Input: part model. Units: mm. Frame: model coordinates. A direction names the side the tool comes from. Coordinates: 2 decimals unless noted, no trailing zeros. Order: outer loops, then holes, each group sorted by start corner. A loop starts at its lowest first (then second) coordinate and runs counter-clockwise, first axis right, second up. Notation, with made-up numbers: M 15,52.25 L 61,52.25 A32 cw 61,81.25 Z; hole C -3.5,69.5 d4. An arc over 180 degrees is marked long. One line per item, written item: value.
Autodesk Inventor part; units mm, degrees
ref_plane "YZ Plane" through (0, 0, 0) normal (1, 0, 0) x (0, 1, 0)
ref_plane "XZ Plane" through (0, 0, 0) normal (0, 1, 0) x (-1, 0, 0)
ref_plane "XY Plane" through (0, 0, 0) normal (0, 0, 1) x (1, 0, 0)
sketch "Skizze1" plane through (0, 0, 0) normal (0, 0, 1) x (1, 0, 0)
  circle A0 centre (0, 0) radius 11.1 construction
  circle A1 centre (0, 0) radius 25
  circle A2 centre (0, 0) radius 15
  circle A3 centre (-15, -15) radius 1.25
  circle A4 centre (15, 15) radius 1.25
  circle A5 centre (15, -15) radius 1.25
  circle A6 centre (-15, 15) radius 1.25
  point P0 (0, 0)
  dimension "d0" = 30
extrude "Extrusion1" add sketch "Skizze1" along normal blind 9 contours A1 | A3 | A4 | A5 | A6
sketch "Skizze2" plane through (0, 0, 9) normal (0, 0, 1) x (1, 0, 0)
  circle A0 centre (0, 0) radius 15
  circle A1 centre (0, 0) radius 25
  point P0 (0, 0)
extrude "Extrusion2" add sketch "Skizze2" against normal blind 2 contours A0
fillet "Rundung1" radius 5 1 edges at (-25, 0, 9)
sketch "Skizze3" plane through (0, 0, 9) normal (0, 0, 1) x (1, 0, 0)
  line L0 (-15, -15) -> (15, -15)
  line L1 (15, -15) -> (15, 15)
  line L2 (15, 15) -> (-15, 15)
  line L3 (-15, 15) -> (-15, -15)
  line L4 (-15, -15) -> (15, 15) construction
  line L5 (15, -15) -> (-15, 15) construction
  point P0 (0, 0)
  dimension "d6" = 30
hole "Bohrung1" at (-15, 15, 9) at (15, 15, 9) at (15, -15, 9) at (-15, -15, 9) direction (0, 0, -1) diameter 3 depth 8 tip angle 118 counterbore diameter 6 counterbore depth 4
properties part number "Cover_G2" material "ABS-Kunststoff"
(1) Cut plane A-A on x = 0. Output: boundary loops of the cut face in (y, z).
Data:
outline: M -25,0 L -15,0 L -15,7 L 15,7 L 15,0 L 25,0 L 25,4 A5 ccw 20,9 L -20,9 A5 ccw -25,4 Z
(2) Access query for faces 1 (the cylindrical face through (-14.985, -0.66, 3.451)), 2 (the cylindrical face through (-12.338, 13.616, 6.528)). Directions: +Z, -Z, +X, -X, +Y, -Y. A direction counts if a zero-diameter tool reaches every point of the face in a straight line with its end or side. Return the directions, or none.
Data:
face 1: -Z
face 2: +Z
(3) Ray query, line 1 (X direction, y = -15.5, z = 5.25); line 2 (X direction, y = 13, z = 6.5); line 3 (X direction, y = 15, z = 7.35). Return the intervals inside material, ascending. Write a range as from..to.
Data:
line 1: x = -19.41..-17.96, -12.04..12.04, 17.96..19.41
line 2: x = -20.57..-17.24, -12.76..-7.48, 7.48..12.76, 17.24..20.57
line 3: x = -18.36..-18, -12..12, 18..18.36
(4) First-contact query: pin 1 (5 mm diameter, centred on x = 20, z = 2.5, fed in from +Y); pin 2 (2.5 mm diameter, centred on x = 15, y = -15, fed in from +Z); pin 3 (5 mm diameter, centred on y = 14.5, z = 7, fed in from +X). Flat tips, straight axial feed; report the tip coordinate or a pass-through.
Data:
pin 1: stops at y = 17.85
pin 2: stops at z = 0.85
pin 3: stops at x = 21.39
(5) Cut plane C-C on z = 6. Output: boundary loops of the cut face in (x, y), plus the area to 3 significant figures.
Data:
outline: C 0,0 d49.17; hole C -15,-15 d6; hole C -15,15 d6; hole C 0,0 d30; hole C 15,-15 d6; hole C 15,15 d6
area: 1,080 mm2
(6) Draft query along X for faces 3 (the flat face through (0, 0, 9)), 4 (the flat face through (-13.7, 13.7, 5)), 5 (the cylindrical face through (23.846, -7.509, 1.972)), 6 (the flat face through (0, 0, 7)). Return one class per face: released by +X, released by -X, zero draft, split by the parting line, or undercut.
Data:
face 3: zero draft
face 4: undercut
face 5: split by the parting line
face 6: undercut
